```python
from build123d import *

# Parameters (mm, degrees)
F0_W      = 10.6066017178
F0_H      = 10.6066017178
F1_DEPTH  = 22.5
F4_DEPTH  = 15
F6_DEPTH  = 15
F9_DEPTH  = 15
F11_DEPTH = 15
F13_DEPTH = 15


# Not quite as in the source:
# - a feature names something its author has since deleted; it is built from what else it names


with BuildPart() as f1:
    # F0 (on Front) → F1 (new body, symmetric)
    with BuildSketch(Plane.XZ):
        Rectangle(F0_W, F0_H)
    extrude(amount=F1_DEPTH, both=True)

    # F3 (on 3pt) → F4 (cut, symmetric)
    with BuildSketch(Plane(origin=(0, 0, 0), x_dir=(0, 1, 0), z_dir=(0.7071067812, 0, -0.7071067812))):
        Polygon((-15, -7.5), (-22.5, 0), (-15, 7.5), (-15, 9.5), (-24.5, 9.5), (-24.5, -9.5), (-15, -9.5), align=None)
        Polygon((15, 7.5), (22.5, 0), (15, -7.5), (15, -9.5), (24.5, -9.5), (24.5, 9.5), (15, 9.5), align=None)
    extrude(amount=F4_DEPTH, both=True, mode=Mode.SUBTRACT)

    # F5 (on 3pt) → F6 (cut, symmetric)
    with BuildSketch(Plane(origin=(0, 0, 0), x_dir=(0, 1, 0), z_dir=(0.7071067812, 0, -0.7071067812))):
        Polygon((7.5, 0), (0, -7.5), (-7.5, 0), (-15, -7.5), (-15, -9.5), (15, -9.5), (15, -7.5), align=None)
    extrude(amount=F6_DEPTH, both=True, mode=Mode.SUBTRACT)

    # F8 (on 3pt) → F9 (cut, symmetric)
    with BuildSketch(Plane(origin=(0, 0, 0), x_dir=(0, -1, 0), z_dir=(-0.7071067812, 0, -0.7071067812))):
        Polygon((-7.5, 7.5), (0, 0), (7.5, 7.5), (7.5, 9.5), (-7.5, 9.5), align=None)
    extrude(amount=F9_DEPTH, both=True, mode=Mode.SUBTRACT)

    # F10 (on 3pt) → F11 (cut, symmetric)
    with BuildSketch(Plane(origin=(0, 0, 0), x_dir=(0, 1, 0), z_dir=(0.7071067812, 0, -0.7071067812))):
        Polygon((-17.0707106781, -9.5), (17.0707106781, -9.5), (7.5, 0.0707106781), (0, -7.4292893219), (-7.5, 0.0707106781), align=None)
    extrude(amount=F11_DEPTH, both=True, mode=Mode.SUBTRACT)

    # F12 (on 3pt) → F13 (cut, symmetric)
    with BuildSketch(Plane(origin=(0, 0, 0), x_dir=(0, -1, 0), z_dir=(-0.7071067812, 0, -0.7071067812))):
        Polygon((9.5707106781, 9.5), (-9.5707106781, 9.5), (0, -0.0707106781), align=None)
    extrude(amount=F13_DEPTH, both=True, mode=Mode.SUBTRACT)


solid = f1.part
```
CAD build for the part. Positions are in the model's coordinates, mm. A direction names the side the tool comes from. Coordinates: 2 decimals unless noted, no trailing zeros. Order: outer loops, then holes, each group sorted by start corner. A loop starts at its lowest first (then second) coordinate and runs counter-clockwise, first axis right, second up. Notation, with made-up numbers: (-9, 29) - (5, 29) arc R34 ccw to (5, 59) - close; hole circle Ø2 at (-22, 27). An arc over 180 degrees is marked (long way). Use a Markdown table: item, result. Add a question column.
(1) Saw through at C-C (y = -4). Give the cut face in (x, z), then the cut area to 3 significant figures.
(2) Flat gauge pins, fed straight in: pin 1 (1.5 mm diameter, centred on x = -1, z = -0.5, fed in from -Y); pin 2 (2 mm diameter, centred on x = 4, y = 17.5, fed in from +Z); pin 3 (2 mm diameter, centred on y = 5, z = 4, fed in from -X). Where does each tip first touch, or does it go through?
(3) Saw through at A-A (z = 1). Give the cut face in (x, y), then the cut area to 3 significant figures.
(4) Drill centre lines: line 1 along Y through (x, z) = (-3.5, 1.5); line 2 along Y through (x, z) = (-0.75, -2.5); line 3 along Y through (x, z) = (-3.5, 2.25). Where is each one in solid material? Low to high. Write a range as [from, to].
(5) Saw through at D-D (x = 2.25). Give the cut face in (y, z), then the cut area to 3 significant figures.
(6) Pull direction Y, two halves, no side cores. Call faces 4 (the face through (2, -19.6, 2.1)), 5 (the face through (5.303, 0, 0)), 6 (the face through (-1.9, 4.6, -2.1)): +Y half, -Y half, draft (parallel to the pull), parting line (faces both ways), or undercut.
(7) Saw through at B-B (x = -3.75). Give the cut face in (y, z).
(8) Which spindle directions (+Z, -Z, +X, -X, +Y, -Y) get a long thin tool onto all of the face, cutting with end or side? Do faces 1 (the face through (-2.024, -2.864, 1.926)), 2 (the face through (1, 0, -5.303)), 3 (the face through (-1.985, 10.483, -2.134)). Say none if no direction does.
Solved:
| question | item | result |
|---|---|---|
| 1 | outline | (-5.2, 0.35) - (0.45, -5.3) - (5.3, -5.3) - (5.3, 5.3) - (-0.25, 5.3) - close |
| 1 | area | 83.2 mm² |
| 2 | pin 1 | stops at y = -22.19 |
| 2 | pin 2 | stops at z = 4.8 |
| 2 | pin 3 | stops at x = -4.7 |
| 3 | outline | (-5.3, -19.46) - (-1, -22.5) - (5.3, -18.04) - (5.3, 18.04) - (-1, 22.5) - (-5.3, 19.46) - (-5.3, 10.61) - (-0.9, 7.5) - (-5.2, 4.46) - (1.1, 0) - (-5.2, -4.46) - (-0.9, -7.5) - (-5.3, -10.61) - close |
| 3 | area | 380 mm² |
| 4 | line 1 | y = [-21.09, -8.98], [-6.02, -3.61], [3.61, 6.02], [8.98, 21.09] |
| 4 | line 2 | y = [-20.2, -9.87], [-5.13, 5.13], [9.87, 20.2] |
| 4 | line 3 | y = [-21.62, -8.45], [-6.55, -4.14], [4.14, 6.55], [8.45, 21.62] |
| 5 | outline | (-22.5, -2.25) - (-20.34, -5.3) - (-9.73, -5.3) - (-7.5, -2.15) - (-5.27, -5.3) - (5.27, -5.3) - (7.5, -2.15) - (9.73, -5.3) - (20.34, -5.3) - (22.5, -2.25) - (17.16, 5.3) - (2.23, 5.3) - (0, 2.15) - (-2.23, 5.3) - (-17.16, 5.3) - close |
| 5 | area | 409 mm² |
| 6 | face 4 | -Y half |
| 6 | face 5 | draft |
| 6 | face 6 | undercut |
| 7 | outline | (-22.5, 3.75) - (-16.1, -5.3) - (-13.97, -5.3) - (-7.5, 3.85) - (-1.03, -5.3) - (1.03, -5.3) - (7.5, 3.85) - (13.97, -5.3) - (16.1, -5.3) - (22.5, 3.75) - (21.4, 5.3) - (6.47, 5.3) - (0, -3.85) - (-6.47, 5.3) - (-21.4, 5.3) - close |
| 8 | face 1 | +Z, -X |
| 8 | face 2 | -Z, +X, -X, +Y, -Y |
| 8 | face 3 | -Z, -X |
